Part model, mm, in its own coordinate system. A direction names the side the tool comes from. Give positions to 0.01 mm unless a question says otherwise; leave off trailing zeros. Order: outer loops, then holes, each group sorted by start corner. A loop starts at its lowest first (then second) coordinate and runs counter-clockwise, first axis right, second up.
1. Drop flat-ended pins along their axis: pin 1 Ø8 at (x, y) = (-54.5, -38.5) entering from +Z; pin 2 Ø10 at (x, y) = (58, -127.5) entering from -Z; pin 3 Ø8 at (x, z) = (176.5, 485.5) entering from +Y. Give the stop position or say it passes through.
2. Slice it at A-A on x = 111. List the corners of the cut face in (y, z).
3. Mould opens along X. For faces 6 (the flat face through (225, -1, 508)), 7 (the flat face through (1, 140, 430)), 8 (the flat face through (190, 174, 677)) say: +X half, -X half, draft (parallel to the pull), parting line (faces both ways), or undercut.
4. Slice it at D-D on z = 771. List the corners of the cut face in (x, y), and give its area (3 significant figures).
5. Slice it at C-C on y = 157. List the corners of the cut face in (x, z), and give its area (3 significant figures).
6. Slice it at B-B on z = 453. List the corners of the cut face in (x, y).
7. Probe line 1 (Y direction, x = 205, z = 340.5); line 2 (Z direction, x = -68.5, y = -188.5); line 3 (Y direction, x = -170, z = 513.5). List the from-to ranges inside material, lowest first.
8. Which spindle directions (+Z, -Z, +X, -X, +Y, -Y) get a long thin tool onto all of the face, cutting with end or side? Do faces 1 (the flat face through (3, -27, 494.97)), 2 (the flat face through (-2.66, 196.814, 865.423)), 3 (the flat face through (3, -45, 544.97)), 4 (the flat face through (-2.66, 206, 939.86)), 5 (the flat face through (190, 157, 210)). Say none if no direction does.
from build123d import *

# Parameters (mm, degrees)
F0_W     = 450
F0_H     = 450
F1_DEPTH = 950
F2_W     = 330
F2_H     = 494.9696660042
F2_W_2   = 50
F2_H_2   = 50
F3_DEPTH = 450.001
F4_W     = 380
F4_H     = 425
F5_DEPTH = 450.001
F6_W     = 380
F6_H     = 275
F6_H_2   = 75
F7_DEPTH = 151.1289788998


with BuildPart() as f1:
    # F0 (on Top) → F1 (new body)
    with BuildSketch(Plane.XY):
        Rectangle(F0_W, F0_H)
    extrude(amount=F1_DEPTH)

    # F2 (on face) → F3 (cut, through all)
    with BuildSketch(Plane.YZ.offset(225)):
        with Locations((-25, 247.4848330021)):
            Rectangle(F2_W, F2_H)
        with Locations((200, 247.4848330021)):
            Rectangle(F2_W_2, F2_H)
        Polygon((225, 950), (175, 544.9696660042), (225, 544.9696660042), align=None)
        with Locations((200, 519.9696660042)):
            Rectangle(F2_W_2, F2_H_2)
        Polygon((-225, 950), (-225, 544.9696660042), (140, 544.9696660042), (190, 950), align=None)
    extrude(amount=-F3_DEPTH, mode=Mode.SUBTRACT)

    # F4 (on face) → F5 (cut, through all)
    with BuildSketch(Plane.XZ.offset(225)):
        with Locations((0, 212.5)):
            Rectangle(F4_W, F4_H)
    extrude(amount=-F5_DEPTH, mode=Mode.SUBTRACT)

    # F6 (on face) → F7 (cut, through all)
    with BuildSketch(Plane(origin=(0, 71.633193695, -8.8429418345), x_dir=(1, 0, 0), z_dir=(0, -0.9924663491, 0.1225175334))):
        with Locations((0, 695.5165094381)):
            Rectangle(F6_W, F6_H)
        with Locations((0, 920.5165094381)):
            Rectangle(F6_W, F6_H_2)
    extrude(amount=-F7_DEPTH, mode=Mode.SUBTRACT)


solid = f1.part
Data:
1. pin 1: stops at z = 544.97
1. pin 2: stops at z = 494.97
1. pin 3: stops at y = 175
2. outline: (-225, 425) - (-190, 425) - (-190, 494.97) - (140, 494.97) - (140, 425) - (175, 425) - (175, 540.65) - (140, 544.97) - (-225, 544.97) - close; (173.69, 817.9) - (208.17, 813.64) - (214.29, 863.27) - (179.82, 867.52) - close; (189.01, 941.96) - (223.48, 937.7) - (225, 950) - (190, 950) - close
3. face 6: +X half
3. face 7: draft
3. face 8: undercut
4. outline: (-225, 167.9) - (-190, 167.9) - (-190, 202.9) - (-225, 202.9) - close; (190, 167.9) - (225, 167.9) - (225, 202.9) - (190, 202.9) - close
4. area: 2,450 mm2
5. outline: (-225, 0) - (-190, 0) - (-190, 425) - (190, 425) - (190, 0) - (225, 0) - (225, 682.68) - (190, 682.68) - (190, 542.87) - (-190, 542.87) - (-190, 682.68) - (-225, 682.68) - close
5. area: 92,600 mm2
6. outline: (-225, -225) - (225, -225) - (225, -190) - (-225, -190) - close; (-225, 140) - (225, 140) - (225, 175) - (-225, 175) - close
7. line 1: y = -225 to -190, 140 to 175
7. line 2: z = 494.97 to 544.97
7. line 3: y = -225 to 175
8. face 1: -Z, +X, -X
8. face 2: +Y
8. face 3: +Z, +X, -X, -Y
8. face 4: -Y
8. face 5: -Z, +Y, -Y
